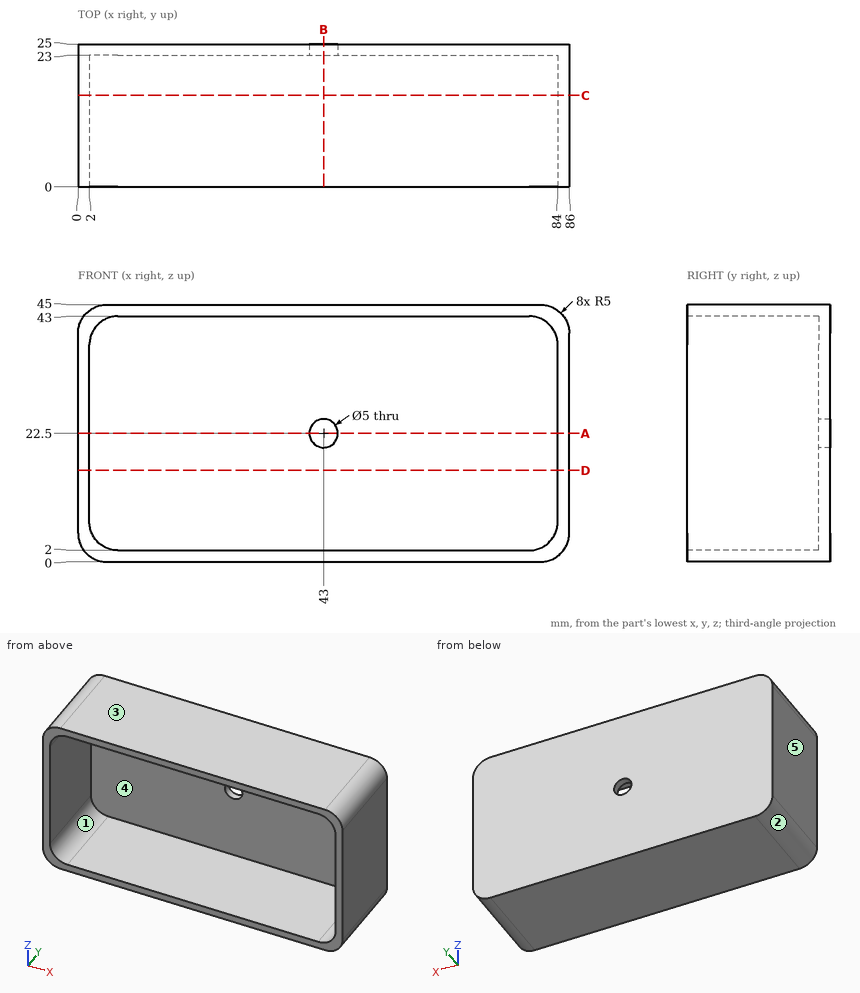
Print and shaded views of the part. All mm, measured from the part's lowest x, y and z. A direction names the side the tool comes from. Round coordinates to 2 decimals unless told otherwise and drop trailing zeros. Order: outer loops, then holes, each group sorted by start corner. A loop starts at its lowest first (then second) coordinate and runs counter-clockwise, first axis right, second up. Notation, with made-up numbers: (74.25, 21) - (95.25, 21) arc R26 ccw to (95.25, 41) - close; hole circle Ø5 at (84, 27). An arc over 180 degrees is marked (long way). Use a Markdown table: item, result.
1) Tool access for the marked faces 1 and 2: list every direction of +Z, -Z, +X, -X, +Y, -Y with a clear straight run to the whole face (end or side of a thin tool).
Recorded:
| item | result |
|---|---|
| face 1 | -Y |
| face 2 | -Z, -X, +Y, -Y |
2) Saw through at D-D on z = 16. Write the cut outline in (x, y).
Recorded:
| item | result |
|---|---|
| outline | (0, 0) - (2, 0) - (2, 23) - (84, 23) - (84, 0) - (86, 0) - (86, 25) - (0, 25) - close |
3) Pull direction Z, two halves, no side cores. Call the marked faces 3, 4 and 5: pulls with the +Z half, pulls with the -Z half, needs draft (parallel to the pull), parting line crosses it, or undercut.
Recorded:
| item | result |
|---|---|
| face 3 | pulls with the +Z half |
| face 4 | undercut |
| face 5 | needs draft |
4) Saw through at A-A on z = 22.5. Write the cut outline in (x, y).
Recorded:
| item | result |
|---|---|
| outline | (0, 0) - (2, 0) - (2, 23) - (40.5, 23) - (40.5, 25) - (0, 25) - close; (45.5, 23) - (84, 23) - (84, 0) - (86, 0) - (86, 25) - (45.5, 25) - close |
5) Flat gauge pin, fed straight in: pin 1 Ø2 at (x, z) = (34, 26) entering from -Y. Where does the tip first touch, or does it go through?
Recorded:
| item | result |
|---|---|
| pin 1 | stops at y = 23 |
6) Saw through at B-B on x = 43. Write the cut outline in (y, z), and give its area (3 significant figures).
Recorded:
| item | result |
|---|---|
| outline | (0, 0) - (25, 0) - (25, 20) - (23, 20) - (23, 2) - (0, 2) - close; (0, 43) - (23, 43) - (23, 25) - (25, 25) - (25, 45) - (0, 45) - close |
| area | 172 mm² |
7) Saw through at C-C on y = 16. Write the cut outline in (x, z), and give its area (3 significant figures).
Recorded:
| item | result |
|---|---|
| outline | (0, 5) arc R5 ccw to (5, 0) - (81, 0) arc R5 ccw to (86, 5) - (86, 40) arc R5 ccw to (81, 45) - (5, 45) arc R5 ccw to (0, 40) - close; hole (2, 7) arc R5 ccw to (7, 2) - (79, 2) arc R5 ccw to (84, 7) - (84, 38) arc R5 ccw to (79, 43) - (7, 43) arc R5 ccw to (2, 38) - close |
| area | 508 mm² |
8) Wall check: L1, parallel to Z at x = 43, y = 23.65; L2, parallel to X at y = 24.45, z = 22.5; L3, parallel to X at y = 10, z = 21.5. Give the ranges that are in metal, low to high.
Recorded:
| item | result |
|---|---|
| L1 | z = 0 to 20, 25 to 45 |
| L2 | x = 0 to 40.5, 45.5 to 86 |
| L3 | x = 0 to 2, 84 to 86 |
